from build123d import *

# Parameters (mm, degrees)
F0_W     = 67.597946
F0_H     = 1.718592
F0_W_2   = 67.025
F0_H_2   = 1.909549
F0_H_3   = 2.5
F1_DEPTH = 5


with BuildPart() as f1:
    # F0 (on Front) → F1 (new body)
    with BuildSketch(Plane.XZ):
        Polygon((54.410804, 59.911989), (-55.589196, 59.911989), (-55.589196, 51.747056), (-4.487936, 51.747056), (-4.487936, 49.247056), (-55.589196, 49.247056), (-55.589196, 41.80489), (-4.487936, 41.80489), (-4.487936, 39.30489), (-55.589196, 39.30489), (-55.589196, 32.05392), (-4.487936, 32.05392), (-4.487936, 29.55392), (-55.589196, 29.55392), (-55.589196, 21.920557), (-4.487936, 21.920557), (-4.487936, 19.420557), (-55.589196, 19.420557), (-55.589196, 11.978389), (-4.487936, 11.978389), (-4.487936, 9.478389), (-55.589196, 9.478389), (-55.589196, 2.5), (-4.487936, 2.5), (-4.487936, 0), (-55.589196, 0), (-55.589196, -6.758772), (-4.487936, -6.758772), (-4.487936, -9.258772), (-55.589196, -9.258772), (-55.589196, -16.499988), (-4.487936, -16.499988), (-4.487936, -18.999988), (-55.589196, -18.999988), (-55.589196, -26.638176), (-4.487936, -26.638176), (-4.487936, -29.120585), (-55.589196, -29.120585), (-55.589196, -35.231136), (-4.487936, -35.231136), (-4.487936, -37.522592), (-55.589196, -37.522592), (-55.589196, -50.088011), (54.410804, -50.088011), (54.410804, -37.522592), (6.205984, -37.522592), (6.205984, -35.231136), (54.410804, -35.231136), (54.410804, -29.120585), (5.156064, -29.120585), (5.156064, -26.620585), (54.410804, -26.620585), (54.410804, -18.999988), (5.156064, -18.999988), (5.156064, -16.499988), (54.410804, -16.499988), (54.410804, -9.258772), (5.156064, -9.258772), (5.156064, -6.758772), (54.410804, -6.758772), (54.410804, 0), (5.156064, 0), (5.156064, 2.5), (54.410804, 2.5), (54.410804, 9.478389), (5.156064, 9.478389), (5.156064, 11.978389), (54.410804, 11.978389), (54.410804, 19.420557), (5.156064, 19.420557), (5.156064, 21.920557), (54.410804, 21.920557), (54.410804, 29.362723), (5.156064, 29.362723), (5.156064, 31.862723), (54.410804, 31.862723), (54.410804, 39.30489), (5.156064, 39.30489), (5.156064, 41.80489), (54.410804, 41.80489), (54.410804, 49.247056), (5.156064, 49.247056), (5.156064, 51.747056), (54.410804, 51.747056), align=None)
        with Locations((5.442537, -41.819068)):
            Rectangle(F0_W, F0_H, mode=Mode.SUBTRACT)
        with Locations((5.156064, -32.17586)):
            Rectangle(F0_W_2, F0_H_2, mode=Mode.SUBTRACT)
        with Locations((5.156064, -22.714809)):
            Rectangle(F0_W_2, F0_H_3, mode=Mode.SUBTRACT)
        with Locations((5.156064, -12.979856)):
            Rectangle(F0_W_2, F0_H_3, mode=Mode.SUBTRACT)
        with Locations((5.156064, -3.037689)):
            Rectangle(F0_W_2, F0_H_3, mode=Mode.SUBTRACT)
        with Locations((5.156064, 6.330893)):
            Rectangle(F0_W_2, F0_H_3, mode=Mode.SUBTRACT)
        with Locations((5.156064, 15.890669)):
            Rectangle(F0_W_2, F0_H_3, mode=Mode.SUBTRACT)
        with Locations((5.156064, 25.832837)):
            Rectangle(F0_W_2, F0_H_3, mode=Mode.SUBTRACT)
        with Locations((5.156064, 35.775003)):
            Rectangle(F0_W_2, F0_H_3, mode=Mode.SUBTRACT)
        with Locations((5.156064, 45.525977)):
            Rectangle(F0_W_2, F0_H_3, mode=Mode.SUBTRACT)
    extrude(amount=F1_DEPTH)


solid = f1.part
Can you work these out from the model? Positions are in its coordinate system, mm. A direction names the side the tool comes from. Coordinates: 2 decimals unless noted, no trailing zeros.
Q1. Which directions (+Z, -Z, +X, -X, +Y, -Y) give clear straight access to the entire face, cutting with the end or side of a thin tool? Please do faces 4 (the face through (-28.356, -2, -3)), 5 (the face through (-30, -2, -19)), 6 (the face through (30, -2, -29.121)).
Results found:
face 4: +Y, -Y
face 5: -X, +Y, -Y
face 6: +X, +Y, -Y
Q2. Please list where these lines run through material, in increasing order: L1, parallel to X at y = -3.2, z = -42; L2, parallel to X at y = -4.7, z = 7; L3, parallel to X at y = -2.7, z = 31.5.
Results found:
L1: x = -55.59 to -28.36, 39.24 to 54.41
L2: x = -55.59 to -28.36, 38.67 to 54.41
L3: x = -4.49 to 5.16
Q3. If we mould it in two halves opening along X, with no side actions, what happens to faces 1 (the face through (54.411, -2, 45)), 2 (the face through (30, -2, -9.259)), 3 (the face through (38.669, -2, 26))? For each: +X half, -X half, draft (parallel to the pull), parting line (faces both ways), or undercut.
Results found:
face 1: +X half
face 2: draft
face 3: undercut
Q4. For P1, Ø8, axis at x = 38, z = -13.5, coming from the +Y side; P2, Ø0.8, axis at y = -3, z = 20.5, coming from the +X side, each with a flat end and sliding along its axis, tell me the tip position at first contact or that it passes through.
Results found:
P1: stops at y = 0
P2: stops at x = 5.16
Q5. Imagine slicing it at A-A, the plane x = 46.5. Count the separate pieces of the cut face and the enclosed holes in it, plus the area to 3 significant figures.
Results found:
separate pieces: 11
enclosed holes: 0
area: 426 mm2
